```python
from build123d import *

# Parameters (mm, degrees)
F1_DEPTH        = 3
F2_DEPTH        = 16
F3_R            = 5
F4_DEPTH        = 14
F5_R            = 4.5
F6_DEPTH        = 16
F7_SIZE         = 1.5
F8_SIZE         = 0.49999
F9_D            = 3.4
F9_CSINK_D      = 6
F9_CSINK_ANGLE  = 90
F10_D           = 3.4
F10_CSINK_D     = 6
F10_CSINK_ANGLE = 90


# Not quite as in the source:
# - a fillet or chamfer is up to 0.001 mm smaller than in the source, because OpenCascade refuses the exact size


with BuildPart() as f1:
    # F0 (on Top) → F1 (new body)
    with BuildSketch(Plane.XY):
        with BuildLine():
            ThreePointArc((9.503875, 3.1106848096), (7.8523539336, 6.1919736516), (5.2411289459, 8.5164879717))
            Line((5.2411289459, 8.5164879717), (-5.2411289459, 8.5164879717))
            ThreePointArc((-5.2411289459, 8.5164879717), (-7.8523539336, 6.1919736516), (-9.503875, 3.1106848096))
            ThreePointArc((-9.503875, 3.1106848096), (-8.5246009554, 2.7831093509), (-7.703875, 2.15645774))
            ThreePointArc((-7.703875, 2.15645774), (0, 8), (7.703875, 2.15645774))
            ThreePointArc((7.703875, 2.15645774), (8.5246009554, 2.7831093509), (9.503875, 3.1106848096))
        make_face()
        with BuildLine():
            ThreePointArc((-7.703875, 2.15645774), (-8.5246009554, 2.7831093509), (-9.503875, 3.1106848096))
            ThreePointArc((-9.503875, 3.1106848096), (-9.705576078, 2.4086911373), (-9.8555, 1.6938476171))
            ThreePointArc((-9.8555, 1.6938476171), (-8.7478718117, 1.149858687), (-8.3, 0))
            ThreePointArc((-8.3, 0), (-8.7478718117, -1.149858687), (-9.8555, -1.6938476171))
            ThreePointArc((-9.8555, -1.6938476171), (-9.705576078, -2.4086911373), (-9.503875, -3.1106848096))
            ThreePointArc((-9.503875, -3.1106848096), (-8.5246009554, -2.7831093509), (-7.703875, -2.15645774))
            ThreePointArc((-7.703875, -2.15645774), (-8, 0), (-7.703875, 2.15645774))
        make_face()
        with BuildLine():
            ThreePointArc((-8.3, 0), (-8.7478718117, 1.149858687), (-9.8555, 1.6938476171))
            ThreePointArc((-9.8555, 1.6938476171), (-10, 0), (-9.8555, -1.6938476171))
            ThreePointArc((-9.8555, -1.6938476171), (-8.7478718117, -1.149858687), (-8.3, 0))
        make_face()
        with BuildLine():
            ThreePointArc((-9.8555, -1.6938476171), (-10, 0), (-9.8555, 1.6938476171))
            ThreePointArc((-9.8555, 1.6938476171), (-11.7, 0), (-9.8555, -1.6938476171))
        make_face()
        with BuildLine():
            ThreePointArc((-9.8555, 1.6938476171), (-9.705576078, 2.4086911373), (-9.503875, 3.1106848096))
            ThreePointArc((-9.503875, 3.1106848096), (-13.15, 0), (-9.503875, -3.1106848096))
            ThreePointArc((-9.503875, -3.1106848096), (-9.705576078, -2.4086911373), (-9.8555, -1.6938476171))
            ThreePointArc((-9.8555, -1.6938476171), (-11.7, 0), (-9.8555, 1.6938476171))
        make_face()
        with BuildLine():
            Line((-5.2411289459, 8.5164879717), (-11.1116800092, 8.5164879717))
            ThreePointArc((-11.1116800092, 8.5164879717), (-13.9999961512, 0.0103809935), (-11.1242977306, -8.5))
            Line((-11.1242977306, -8.5), (-5.2678268764, -8.5))
            ThreePointArc((-5.2678268764, -8.5), (-7.8620591219, -6.1796461357), (-9.503875, -3.1106848096))
            ThreePointArc((-9.503875, -3.1106848096), (-13.15, 0), (-9.503875, 3.1106848096))
            ThreePointArc((-9.503875, 3.1106848096), (-7.8523539336, 6.1919736516), (-5.2411289459, 8.5164879717))
        make_face()
        with BuildLine():
            ThreePointArc((11.1242977306, -8.5), (13.2616018683, -4.486637481), (14, 0))
            ThreePointArc((14, 0), (13.258271383, 4.4964697192), (11.1116800092, 8.5164879717))
            Line((11.1116800092, 8.5164879717), (5.2411289459, 8.5164879717))
            ThreePointArc((5.2411289459, 8.5164879717), (7.8523539336, 6.1919736516), (9.503875, 3.1106848096))
            ThreePointArc((9.503875, 3.1106848096), (12.0444689103, 2.3963820386), (13.15, 0))
            ThreePointArc((13.15, 0), (12.0444689103, -2.3963820386), (9.503875, -3.1106848096))
            ThreePointArc((9.503875, -3.1106848096), (7.8620591219, -6.1796461357), (5.2678268764, -8.5))
            Line((5.2678268764, -8.5), (11.1242977306, -8.5))
        make_face()
        with BuildLine():
            ThreePointArc((11.7, 0), (11.149858687, 1.2521281883), (9.8555, 1.6938476171))
            ThreePointArc((9.8555, 1.6938476171), (9.9638095124, 0.85), (10, 0))
            ThreePointArc((10, 0), (9.9638095124, -0.85), (9.8555, -1.6938476171))
            ThreePointArc((9.8555, -1.6938476171), (11.149858687, -1.2521281883), (11.7, 0))
        make_face()
        with BuildLine():
            ThreePointArc((13.15, 0), (12.0444689103, 2.3963820386), (9.503875, 3.1106848096))
            ThreePointArc((9.503875, 3.1106848096), (9.705576078, 2.4086911373), (9.8555, 1.6938476171))
            ThreePointArc((9.8555, 1.6938476171), (11.149858687, 1.2521281883), (11.7, 0))
            ThreePointArc((11.7, 0), (11.149858687, -1.2521281883), (9.8555, -1.6938476171))
            ThreePointArc((9.8555, -1.6938476171), (9.705576078, -2.4086911373), (9.503875, -3.1106848096))
            ThreePointArc((9.503875, -3.1106848096), (12.0444689103, -2.3963820386), (13.15, 0))
        make_face()
        with BuildLine():
            ThreePointArc((10, 0), (9.9638095124, 0.85), (9.8555, 1.6938476171))
            ThreePointArc((9.8555, 1.6938476171), (8.3, 0), (9.8555, -1.6938476171))
            ThreePointArc((9.8555, -1.6938476171), (9.9638095124, -0.85), (10, 0))
        make_face()
        with BuildLine():
            ThreePointArc((9.8555, 1.6938476171), (9.705576078, 2.4086911373), (9.503875, 3.1106848096))
            ThreePointArc((9.503875, 3.1106848096), (8.5246009554, 2.7831093509), (7.703875, 2.15645774))
            ThreePointArc((7.703875, 2.15645774), (7.9256230039, 1.088347371), (8, 0))
            ThreePointArc((8, 0), (7.9256230039, -1.088347371), (7.703875, -2.15645774))
            ThreePointArc((7.703875, -2.15645774), (8.5246009554, -2.7831093509), (9.503875, -3.1106848096))
            ThreePointArc((9.503875, -3.1106848096), (9.705576078, -2.4086911373), (9.8555, -1.6938476171))
            ThreePointArc((9.8555, -1.6938476171), (8.3, 0), (9.8555, 1.6938476171))
        make_face()
        with BuildLine():
            Line((-5.2678268764, -8.5), (5.2678268764, -8.5))
            ThreePointArc((5.2678268764, -8.5), (7.8620591219, -6.1796461357), (9.503875, -3.1106848096))
            ThreePointArc((9.503875, -3.1106848096), (8.5246009554, -2.7831093509), (7.703875, -2.15645774))
            ThreePointArc((7.703875, -2.15645774), (0, -8), (-7.703875, -2.15645774))
            ThreePointArc((-7.703875, -2.15645774), (-8.5246009554, -2.7831093509), (-9.503875, -3.1106848096))
            ThreePointArc((-9.503875, -3.1106848096), (-7.8620591219, -6.1796461357), (-5.2678268764, -8.5))
        make_face()
        with BuildLine():
            ThreePointArc((7.703875, -2.15645774), (6.85, 0), (7.703875, 2.15645774))
            ThreePointArc((7.703875, 2.15645774), (0, 8), (-7.703875, 2.15645774))
            ThreePointArc((-7.703875, 2.15645774), (-7.0712379962, 1.1596780264), (-6.85, 0))
            ThreePointArc((-6.85, 0), (-7.0712379962, -1.1596780264), (-7.703875, -2.15645774))
            ThreePointArc((-7.703875, -2.15645774), (0, -8), (7.703875, -2.15645774))
        make_face()
        with BuildLine():
            ThreePointArc((8, 0), (7.9256230039, 1.088347371), (7.703875, 2.15645774))
            ThreePointArc((7.703875, 2.15645774), (6.85, 0), (7.703875, -2.15645774))
            ThreePointArc((7.703875, -2.15645774), (7.9256230039, -1.088347371), (8, 0))
        make_face()
        with BuildLine():
            ThreePointArc((-6.85, 0), (-7.0712379962, 1.1596780264), (-7.703875, 2.15645774))
            ThreePointArc((-7.703875, 2.15645774), (-8, 0), (-7.703875, -2.15645774))
            ThreePointArc((-7.703875, -2.15645774), (-7.0712379962, -1.1596780264), (-6.85, 0))
        make_face()
    extrude(amount=F1_DEPTH)

    # F0 (on Top) → F2 (join)
    with BuildSketch(Plane.XY):
        with BuildLine():
            ThreePointArc((7.703875, -2.15645774), (6.85, 0), (7.703875, 2.15645774))
            ThreePointArc((7.703875, 2.15645774), (0, 8), (-7.703875, 2.15645774))
            ThreePointArc((-7.703875, 2.15645774), (-7.0712379962, 1.1596780264), (-6.85, 0))
            ThreePointArc((-6.85, 0), (-7.0712379962, -1.1596780264), (-7.703875, -2.15645774))
            ThreePointArc((-7.703875, -2.15645774), (0, -8), (7.703875, -2.15645774))
        make_face()
        with BuildLine():
            ThreePointArc((-6.85, 0), (-7.0712379962, 1.1596780264), (-7.703875, 2.15645774))
            ThreePointArc((-7.703875, 2.15645774), (-8, 0), (-7.703875, -2.15645774))
            ThreePointArc((-7.703875, -2.15645774), (-7.0712379962, -1.1596780264), (-6.85, 0))
        make_face()
        with BuildLine():
            ThreePointArc((8, 0), (7.9256230039, 1.088347371), (7.703875, 2.15645774))
            ThreePointArc((7.703875, 2.15645774), (6.85, 0), (7.703875, -2.15645774))
            ThreePointArc((7.703875, -2.15645774), (7.9256230039, -1.088347371), (8, 0))
        make_face()
    extrude(amount=F2_DEPTH)

    # F3 (on face) → F4 (join)
    with BuildSketch(Plane.XY.offset(16)):
        Circle(F3_R)
    extrude(amount=F4_DEPTH)

    # F5 (on face) → F6 (join)
    with BuildSketch(Plane.XY.offset(30)):
        Circle(F5_R)
    extrude(amount=F6_DEPTH)

    # F7
    f7_edges = [f1.edges().sort_by_distance(p)[0] for p in [
        (-4.5, 0, 46),
    ]]
    chamfer(f7_edges, length=F7_SIZE)

    # F8 (size 0.5 in the source; OpenCascade refuses exactly that, so slightly less here)
    f8_edges = [f1.edges().sort_by_distance(p)[0] for p in [
        (-7.703875, 2.156458, 16),
        (-5, 0, 30),
    ]]
    chamfer(f8_edges, length=F8_SIZE)

    # F9 (through all)
    with Locations(Plane(origin=(0, 0, 0), x_dir=(1, 0, 0), z_dir=(0, 0, -1))):
        with Locations((10, 0)):
            CounterSinkHole(F9_D / 2, F9_CSINK_D / 2, counter_sink_angle=F9_CSINK_ANGLE)

    # F10 (through all)
    with Locations(Plane(origin=(0, 0, 0), x_dir=(1, 0, 0), z_dir=(0, 0, -1))):
        with Locations((-10, 0)):
            CounterSinkHole(F10_D / 2, F10_CSINK_D / 2, counter_sink_angle=F10_CSINK_ANGLE)


solid = f1.part
```
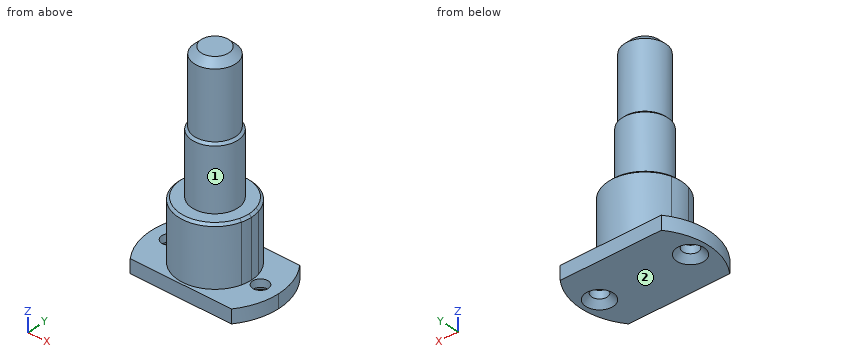
Build history of the part. All positions in model axes, mm. Face numbers are marked on the shaded views. A direction names the side the tool comes from. Round coordinates to 2 decimals unless told otherwise and drop trailing zeros. Write each loop counter-clockwise with the first axis right and the second up, starting at its lowest first coordinate (ties: lowest second). Pieces come first, ordered by that corner, then holes.
1) Band-saw the part on C-C, the plane z = 15. List the corners of the cut face in (x, y).
2) 3-axis set-ups, long thin cutter, end or side, ignore diameter. For the marked faces 1 and 2: which of +Z, -Z, +X, -X, +Y, -Y reach the whole face in a straight line?
3) Band-saw the part on D-D, the plane z = 32. List the corners of the cut face in (x, y), and give its area (3 significant figures).
4) Pin check, flat tips, straight feed: pin 1 (3 mm diameter, centred on x = -5, z = 20.5, fed in from -Y); pin 2 (8 mm diameter, centred on x = 9, y = 3.5, fed in from +Z); pin 3 (4 mm diameter, centred on y = -3.5, z = 40.5, fed in from -X). Stop position of each tip, or through.
5) Band-saw the part on A-A, the plane x = -10. List the corners of the cut face in (y, z).
6) Drill centre lines: probe 1 along Z at (x, y) = (-7.25, 5.75); probe 2 along Z at (x, y) = (-5.25, 2.5); probe 3 along X at (y, z) = (-2.75, 12). Where is each one in solid material? Low to high.
Ans:
1. outline: circle Ø16 at (0, 0)
2. face 1: +Z
2. face 2: -Z, +X, -X, +Y, -Y
3. outline: circle Ø9 at (0, 0)
3. area: 63.6 mm2
4. pin 1: stops at y = -3.57
4. pin 2: stops at z = 16
4. pin 3: stops at x = -4.24
5. outline: (-8.5, 0) - (-3, 0) - (-1.7, 1.3) - (-1.7, 3) - (-8.5, 3) - close; (1.7, 1.3) - (3, 0) - (8.52, 0) - (8.52, 3) - (1.7, 3) - close
6. probe 1: z = 0 to 3
6. probe 2: z = 0 to 16
6. probe 3: x = -7.51 to 7.51
